from build123d import *

# Parameters (mm, degrees)
F0_W     = 80
F0_H     = 50
F1_DEPTH = 12.5
F2_T     = -2.5
F3_R     = 2
F4_R     = 2
F6_DEPTH = 2


with BuildPart() as f1:
    # F0 (on Front) → F1 (new body, symmetric)
    with BuildSketch(Plane.XZ):
        Rectangle(F0_W, F0_H)
    extrude(amount=F1_DEPTH, both=True)

    # F2
    f2_openings = [f1.faces().sort_by_distance(p)[0] for p in [
        (0, -12.5, 0),
    ]]
    offset(amount=F2_T, openings=f2_openings)

    # F3
    f3_edges = [f1.edges().sort_by_distance(p)[0] for p in [
        (37.5, 10, 0),
        (0, 10, 22.5),
        (37.5, -1.25, 22.5),
        (37.5, -1.25, -22.5),
        (-37.5, -1.25, -22.5),
        (0, 10, -22.5),
        (-37.5, 10, 0),
        (-37.5, -1.25, 22.5),
    ]]
    fillet(f3_edges, radius=F3_R)

    # F4
    f4_edges = [f1.edges().sort_by_distance(p)[0] for p in [
        (0, 12.5, 25),
        (-40, 12.5, 0),
        (0, 12.5, -25),
        (40, 12.5, 0),
        (-40, 0, 25),
        (40, 0, 25),
        (-40, 0, -25),
        (40, 0, -25),
    ]]
    fillet(f4_edges, radius=F4_R)

    # F5 (on face) → F6 (cut)
    with BuildSketch(Plane.XZ.offset(12.5)):
        with BuildLine():
            Line((38, 24), (-38, 24))
            ThreePointArc((-38, 24), (-38.7071067812, 23.7071067812), (-39, 23))
            Line((-39, 23), (-39, -23))
            ThreePointArc((-39, -23), (-38.7071067812, -23.7071067812), (-38, -24))
            Line((-38, -24), (38, -24))
            ThreePointArc((38, -24), (38.7071067812, -23.7071067812), (39, -23))
            Line((39, -23), (39, 23))
            ThreePointArc((39, 23), (38.7071067812, 23.7071067812), (38, 24))
        make_face()
    extrude(amount=-F6_DEPTH, mode=Mode.SUBTRACT)


solid = f1.part
The listing builds one solid part. Answer for the finished solid, in the listing's coordinates (mm). A direction names the side the tool comes from. Round coordinates to 2 decimals unless told otherwise and drop trailing zeros. Write each loop counter-clockwise with the first axis right and the second up, starting at its lowest first coordinate (ties: lowest second). Pieces come first, ordered by that corner, then holes. Notation, with made-up numbers: (48.25, 37) - (96.25, 37) arc R19 ccw to (96.25, 73) - close; hole circle Ø7 at (17, -27.5). An arc over 180 degrees is marked (long way). Use a Markdown table: item, result. Add a question column.
1. The part is cut by section C-C (x = -20). Write down the section's boundary in (y, z).
2. Consider line 1 (Z direction, x = 5.5, y = -5.25); line 2 (X direction, y = -5, z = -6.5); line 3 (Y direction, x = 27.5, z = 9). Determine where each line is inside the solid, lowest interval first.
3. The part is cut by section B-B (z = 10). Write down the section's boundary in (x, y).
4. A tool of negligible diameter and unlimited length cuts with its end or side. For faces 5 (the face through (-0.5, 9.4, -21.93)), 6 (the face through (40, -1, 0)), from which of +Z, -Z, +X, -X, +Y, -Y can it reach the whole face along a straight path? Write none if from no direction.
5. For a pull along Z with two mould halves and no side action, classify faces 1 (the face through (-39.43, -0.84, 24.4)), 2 (the face through (39, -12, 0)), 3 (the face through (0, 10, 0)), 4 (the face through (39.43, 11.9, 0.32)) as +Z half, -Z half, draft (parallel to the pull), parting line (faces both ways), or undercut.
6. The part is cut by section A-A (y = -0.5). Write down the section's boundary in (x, z), and give its area (3 significant figures).
7. A flat-ended cylindrical pin translates along its axis: P1, Ø12.5, axis at x = 3, z = -4, coming from the -Y side. Find the tip coordinate at first contact, or state that the pin passes through.
Reported:
| question | item | result |
|---|---|---|
| 1 | outline | (-12.5, -25) - (10.5, -25) arc R2 ccw to (12.5, -23) - (12.5, 23) arc R2 ccw to (10.5, 25) - (-12.5, 25) - (-12.5, 24) - (-10.5, 24) - (-10.5, 22.5) - (8, 22.5) arc R2 cw to (10, 20.5) - (10, -20.5) arc R2 cw to (8, -22.5) - (-10.5, -22.5) - (-10.5, -24) - (-12.5, -24) - close |
| 2 | line 1 | -25 to -22.5, 22.5 to 25 |
| 2 | line 2 | -40 to -37.5, 37.5 to 40 |
| 2 | line 3 | 10 to 12.5 |
| 3 | outline | (-40, -12.5) - (-39, -12.5) - (-39, -10.5) - (-37.5, -10.5) - (-37.5, 8) arc R2 cw to (-35.5, 10) - (35.5, 10) arc R2 cw to (37.5, 8) - (37.5, -10.5) - (39, -10.5) - (39, -12.5) - (40, -12.5) - (40, 10.5) arc R2 ccw to (38, 12.5) - (-38, 12.5) arc R2 ccw to (-40, 10.5) - close |
| 4 | face 5 | -Y |
| 4 | face 6 | +Z, -Z, +X, +Y, -Y |
| 5 | face 1 | +Z half |
| 5 | face 2 | undercut |
| 5 | face 3 | undercut |
| 5 | face 4 | draft |
| 6 | outline | (-40, -23) arc R2 ccw to (-38, -25) - (38, -25) arc R2 ccw to (40, -23) - (40, 23) arc R2 ccw to (38, 25) - (-38, 25) arc R2 ccw to (-40, 23) - close; hole (-37.5, -20.5) arc R2 ccw to (-35.5, -22.5) - (35.5, -22.5) arc R2 ccw to (37.5, -20.5) - (37.5, 20.5) arc R2 ccw to (35.5, 22.5) - (-35.5, 22.5) arc R2 ccw to (-37.5, 20.5) - close |
| 6 | area | 625 mm^2 |
| 7 | P1 | y = 10 |
